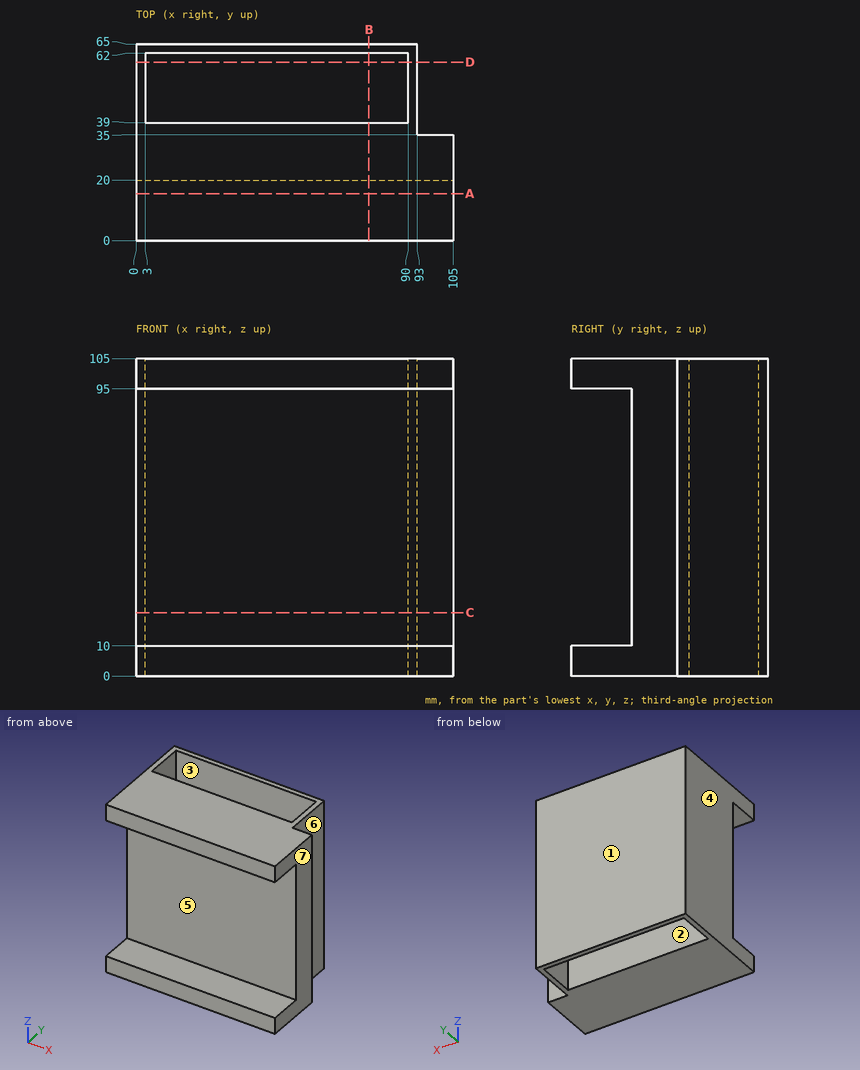
For this review, use the dimensioned drawing (mm, ordinates from the lowest corner) and the shaded views. A direction names the side the tool comes from. Coordinates: 2 decimals unless noted, no trailing zeros. Loops run counter-clockwise (first coordinate to the right, second up) from the corner with the lowest first, then second, coordinate; pieces in that order, holes last.
1. Mouldability with a two-part tool opening along Y and no side actions: class the marked faces 1, 2, 3 and 4 as +Y half, -Y half, draft (parallel to the pull), parting line (faces both ways), or undercut.
2. Add section A-A, the plane y = 15.5. Give the boundary of the cut face in (x, z), then the cut area to 3 significant figures.
3. Add section B-B, the plane x = 77. Give the boundary of the cut face in (y, z), then the cut area to 3 significant figures.
4. For line 1 (Y direction, x = 58.5, z = 32.5); line 2 (X direction, y = 41.5, z = 81); line 3 (Y direction, x = 7.5, z = 8.5), list the stretches that pass through material, from the lowest coordinate up.
5. Insertion check: P1, Ø18.5, axis at y = 51, z = 67, coming from the +X side; P2, Ø3.5, axis at x = 99.5, z = 78.5, coming from the +Y side; P3, Ø12, axis at x = 72.5, z = 31.5, coming from the -Y side. Each pin has a flat end and moves straight along its axis. Give the tip position at first contact, or say it passes through.
6. Add section D-D, the plane y = 59. Give the boundary of the cut face in (x, z), then the cut area to 3 significant figures.
7. For the marked faces 5, 6 and 7, list the 3-axis set-ups (+Z, -Z, +X, -X, +Y, -Y) from which the entire face can be reached by the end or side of a thin tool; tool diameter is ignored.
8. Add section C-C, the plane z = 21. Give the boundary of the cut face in (x, y), then the cut area to 3 significant figures.
Result:
1. face 1: +Y half
1. face 2: undercut
1. face 3: undercut
1. face 4: draft
2. outline: (0, 0) - (105, 0) - (105, 10) - (0, 10) - close; (0, 95) - (105, 95) - (105, 105) - (0, 105) - close
2. area: 2,100 mm2
3. outline: (0, 0) - (39, 0) - (39, 105) - (0, 105) - (0, 95) - (20, 95) - (20, 10) - (0, 10) - close; (62, 0) - (65, 0) - (65, 105) - (62, 105) - close
3. area: 2,710 mm2
4. line 1: y = 20 to 39, 62 to 65
4. line 2: x = 0 to 3, 90 to 93
4. line 3: y = 0 to 39, 62 to 65
5. P1: stops at x = 93
5. P2: stops at y = 35
5. P3: stops at y = 20
6. outline: (0, 0) - (3, 0) - (3, 105) - (0, 105) - close; (90, 0) - (93, 0) - (93, 105) - (90, 105) - close
6. area: 630 mm2
7. face 5: +X, -X, -Y
7. face 6: +Z, -Z, +X, +Y
7. face 7: +Z, -Z, +X, +Y, -Y
8. outline: (0, 20) - (105, 20) - (105, 35) - (93, 35) - (93, 65) - (0, 65) - close; hole (3, 39) - (90, 39) - (90, 62) - (3, 62) - close
8. area: 2,360 mm2
